```python
from build123d import *

# Parameters (mm, degrees)
F1_DEPTH = 2.54
F2_SIZE  = 2.032
F3_R     = 1.400292
F4_R     = 1.388776


with BuildPart() as f1:
    # F0 (on Top) → F1 (new body)
    with BuildSketch(Plane.XY):
        Polygon((3.175, 11.1125), (3.175, 14.9225), (-3.175, 14.9225), (-3.175, -14.9225), (0, -14.9225), (0, 1.5875), (3.175, 1.5875), (3.175, 4.7625), (0, 4.7625), (0, 11.1125), align=None)
    extrude(amount=F1_DEPTH)

    # F2
    f2_edges = [f1.edges().sort_by_distance(p)[0] for p in [
        (3.175, 1.5875, 1.27),
        (3.175, 14.9225, 1.27),
        (-3.175, 14.9225, 1.27),
    ]]
    chamfer(f2_edges, length=F2_SIZE)

    # F3
    f3_edges = [f1.edges().sort_by_distance(p)[0] for p in [
        (0, -14.9225, 1.27),
    ]]
    fillet(f3_edges, radius=F3_R)

    # F4
    f4_edges = [f1.edges().sort_by_distance(p)[0] for p in [
        (-3.175, -14.9225, 1.27),
    ]]
    fillet(f4_edges, radius=F4_R)


solid = f1.part
```
CAD build for the part. Positions are in the model's coordinates, mm. A direction names the side the tool comes from. Coordinates: 2 decimals unless noted, no trailing zeros. Write each loop counter-clockwise with the first axis right and the second up, starting at its lowest first coordinate (ties: lowest second). Pieces come first, ordered by that corner, then holes. Notation, with made-up numbers: (24, 75) -> (34, 75) arc R6 cw to (34, 83) -> close; hole circle Ø5 at (86, 33.25). An arc over 180 degrees is marked (long way). Use CSV: the item, a comma, the result in double quotes. Start each with the question number.
Item 1: Tool access for faces 1 (the flat face through (0, -6, 1)), 2 (the flat face through (0, 8, 1)), 3 (the flat face through (-1, 0, 0)): list every direction of +Z, -Z, +X, -X, +Y, -Y with a clear straight run to the whole face (end or side of a thin tool).
Item 2: Two-plate mould, pull along Y, no slides. Class faces 4 (the flat face through (0.6, 1.588, 1.3)), 5 (the flat face through (2.145, 13.921, 1.252)), 6 (the flat face through (2, 4.762, 1)): +Y half, -Y half, draft (parallel to the pull), parting line (faces both ways), or undercut.
Item 3: Band-saw the part on A-A, the plane x = 1.75. Write the cut outline in (y, z), plus the area to 3 significant figures.
Item 4: Wall check: probe 1 along Y at (x, z) = (0.75, 2.3); probe 2 along X at (y, z) = (10.25, 0.45) (3 decimals); probe 3 along Y at (x, z) = (1.5, 2.3). Give the ranges that are in metal, low to high.
Item 5: Band-saw the part on C-C, the plane y = -7. Write the cut outline in (x, z) (3 decimals).
Item 6: Band-saw the part on D-D, the plane x = -2.5. Write the cut outline in (y, z).
Response values:
1,face 1,"+Z, -Z, +X, -Y"
1,face 2,"+Z, -Z, +X"
1,face 3,"-Z, +X, -X, +Y, -Y"
2,face 4,"-Y half"
2,face 5,"+Y half"
2,face 6,"undercut"
3,outline,"(2.19, 0) -> (4.76, 0) -> (4.76, 2.54) -> (2.19, 2.54) -> close; (11.11, 0) -> (14.32, 0) -> (14.32, 2.54) -> (11.11, 2.54) -> close"
3,area,"14.7 mm2"
4,probe 1,"y = 1.59 to 4.76, 11.11 to 14.92"
4,probe 2,"x = -3.175 to 0"
4,probe 3,"y = 1.94 to 4.76, 11.11 to 14.57"
5,outline,"(-3.175, 0) -> (0, 0) -> (0, 2.54) -> (-3.175, 2.54) -> close"
6,outline,"(-14.73, 0) -> (13.57, 0) -> (13.57, 2.54) -> (-14.73, 2.54) -> close"
